Geometry: see drawing. Coordinates: mm, zero at the bounding-box minimum. A direction names the side the tool comes from. Coordinates: 2 decimals unless noted, no trailing zeros. Write each loop counter-clockwise with the first axis right and the second up, starting at its lowest first coordinate (ties: lowest second). Pieces come first, ordered by that corner, then holes. Notation, with made-up numbers: (64.5, 28.5) - (106.5, 28.5) arc R14 cw to (106.5, 45.5) - close; hole circle Ø10 at (66.25, -29.75). An arc over 180 degrees is marked (long way). One line per question, with ' | ' between items. Start each with the question number.
Q1. Cut plane B-B, the plane x = 22.5. Return loops of the section in (y, z), plus the area to 3 significant figures.
Q2. Line query: line 1 (Z direction, x = 37, y = 20); line 2 (X direction, y = 10, z = 9); line 3 (X direction, y = 4, z = 38.5). Output: solid intervals per line, ascending.
Q3. Cut plane A-A, the plane y = 9.5. Return loops of the section in (x, z), plus the area to 3 significant figures.
Q4. Access query for the marked faces 1, 2 and 3. Directions: +Z, -Z, +X, -X, +Y, -Y. A direction counts if a zero-diameter tool reaches every point of the face in a straight line with its end or side. Return the directions, or none.
Q5. Contact query for flat-ended pins moving along their axis: P1, Ø1.5, axis at x = 44.5, y = 8, coming from the -Z side; P2, Ø12.5, axis at y = 14.5, z = 12.5, coming from the -X side; P3, Ø6, axis at y = 22, z = 54, coming from the -X side. Output: stop coordinate, or through.
Q6. Cut plane C-C, the plane z = 67. Return loops of the section in (x, y), plus the area to 3 significant figures.
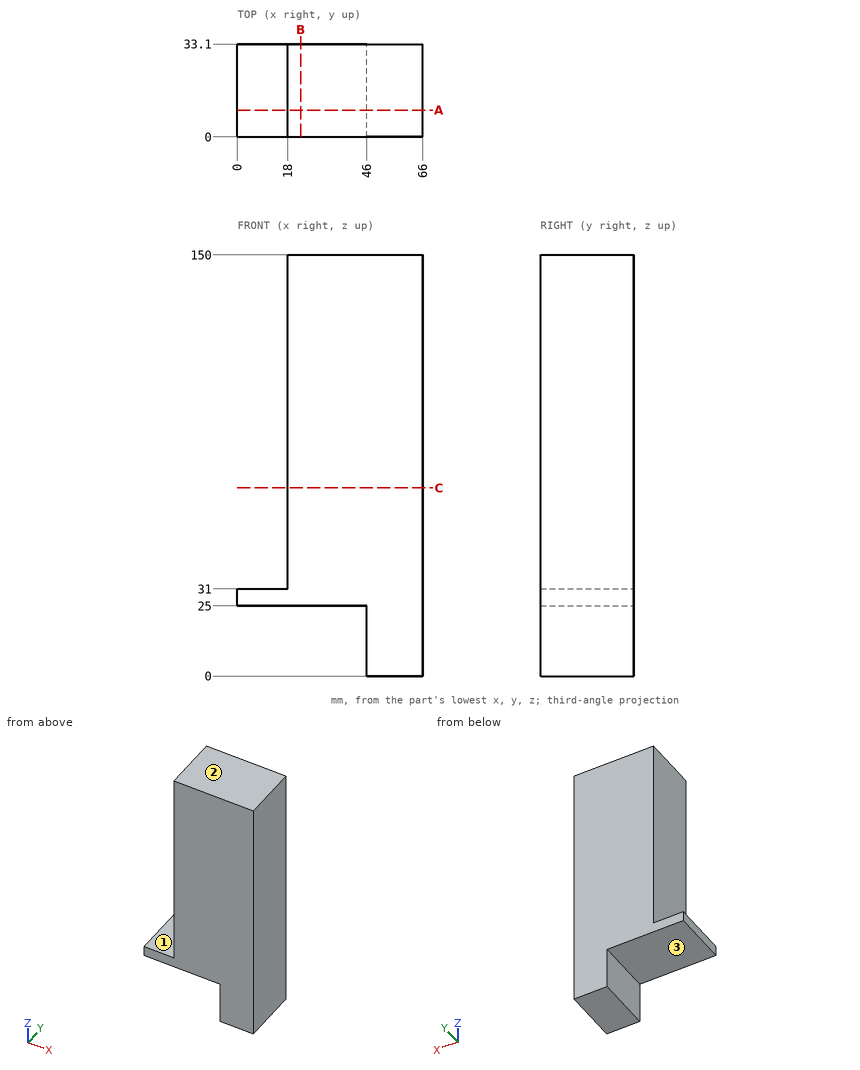
Reply:
1) outline: (0, 25) - (33.1, 25) - (33.1, 150) - (0, 150) - close | area: 4,140 mm^2
2) line 1: z = 25 to 150 | line 2: x = 46 to 66 | line 3: x = 18 to 66
3) outline: (0, 25) - (46, 25) - (46, 0) - (66, 0) - (66, 150) - (18, 150) - (18, 31) - (0, 31) - close | area: 6,610 mm^2
4) face 1: +Z, -X, +Y, -Y | face 2: +Z, +X, -X, +Y, -Y | face 3: -Z, -X, +Y, -Y
5) P1: stops at z = 25 | P2: stops at x = 46 | P3: stops at x = 18
6) outline: (18, 0) - (66, 0) - (66, 33.1) - (18, 33.1) - close | area: 1,590 mm^2
